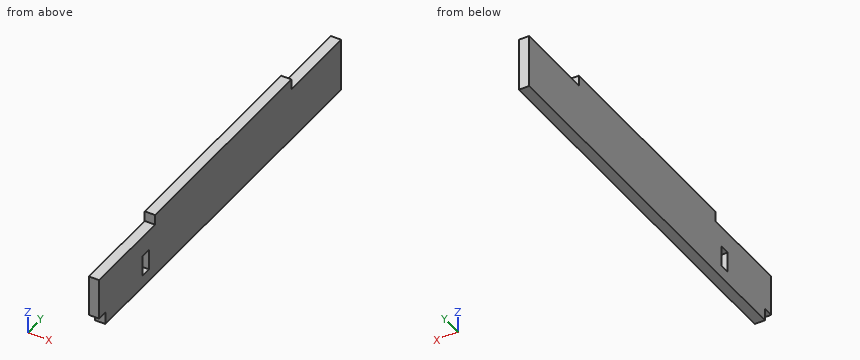
Autodesk Inventor part; units mm, degrees
ref_plane "YZ Plane" through (0, 0, 0) normal (1, 0, 0) x (0, 1, 0)
ref_plane "XZ Plane" through (0, 0, 0) normal (0, 1, 0) x (-1, 0, 0)
ref_plane "XY Plane" through (0, 0, 0) normal (0, 0, 1) x (1, 0, 0)
sketch "Sketch1" plane through (0, 0, 0) normal (1, 0, 0) x (0, 1, 0)
  line L0 (0, 0) -> (200, 0)
  line L1 (200, 0) -> (200, 31)
  line L2 (200, 31) -> (0, 31)
  line L3 (0, 31) -> (0, 0)
  dimension "d0" = 31
  dimension "d1" = 200
extrude "Extrusion1" add sketch "Sketch1" along normal blind 5
sketch "Sketch2" plane through (0, 0, 0) normal (-1, 0, 0) x (0, 0, 1)
  line L0 (0, 200) -> (31, 200)
  line L1 (31, 200) -> (26, 200)
  line L2 (26, 200) -> (26, 195)
  line L3 (26, 195) -> (31, 195)
  line L4 (31, 195) -> (31, 200)
  line L5 (0, 200) -> (5, 200)
  line L6 (5, 200) -> (5, 195)
  line L7 (5, 195) -> (0, 195)
  line L8 (0, 195) -> (0, 200)
  line L9 (31, 0) -> (0, 0)
  line L10 (0, 0) -> (5, 0)
  line L11 (5, 0) -> (5, 5)
  line L12 (5, 5) -> (0, 5)
  line L13 (0, 5) -> (0, 0)
  line L14 (31, 200) -> (31, 0)
  line L15 (31, 0) -> (26, 0)
  line L16 (26, 0) -> (26, 5)
  line L17 (26, 5) -> (31, 5)
  line L18 (31, 5) -> (31, 0)
  line L19 (31, 195) -> (26, 195)
  line L20 (26, 195) -> (26, 155)
  line L21 (26, 155) -> (31, 155)
  line L22 (31, 155) -> (31, 195)
  line L23 (31, 5) -> (26, 5)
  line L24 (26, 5) -> (26, 45)
  line L25 (26, 45) -> (31, 45)
  line L26 (31, 45) -> (31, 5)
  point P0 (31, 5)
  point P1 (26, 0)
  point P2 (31, 45)
  point P3 (31, 155)
  dimension "d4" = 5
  dimension "d5" = 5
  dimension "d6" = 5
  dimension "d7" = 5
  dimension "d8" = 5
  dimension "d9" = 5
  dimension "d10" = 5
  dimension "d11" = 5
  dimension "d14" = 40
  dimension "d15" = 40
extrude "Extrusion2" cut sketch "Sketch2" against normal blind 10 contours L0 L4 L3 L2 | L3 L14 L21 L20 | L9 L16 L17 L14 | L17 L24 L25 L14
sketch "Sketch3" plane through (0, 0, 0) normal (-1, 0, 0) x (0, 0, 1)
  line L0 (6, 35) -> (16, 35)
  line L1 (6, 40) -> (16, 40)
  line L2 (1, 40) -> (1, 35)
  line L3 (16, 40) -> (16, 35)
  line L4 (26, 45) -> (26, 0)
  point P0 (0, 0)
  point P1 (26, 0)
sketch "Sketch3 outline for Extrusion3" plane through (0, 0, 0) normal (-1, 0, 0) x (0, 0, 1)
  line L0 (6, 40) -> (6, 35)
  line L1 (16, 40) -> (6, 40)
  line L2 (16, 35) -> (16, 40)
  line L3 (6, 35) -> (16, 35)
extrude "Extrusion3" cut sketch "Sketch3 outline for Extrusion3" against normal blind 10
sketch "Sketch4" plane through (0, 0, 0) normal (-1, 0, 0) x (0, 0, 1)
  line L0 (26, 200) -> (26, 155)
  line L1 (0, 0) -> (0, 200)
  line L2 (26, 200) -> (0, 200)
  line L3 (0, 200) -> (0, 195)
  line L4 (0, 195) -> (26, 195)
  line L5 (26, 195) -> (26, 200)
  dimension "d18" = 5
extrude "Extrusion4" cut sketch "Sketch4" against normal blind 10
sketch "Sketch5" plane through (5, 0, 0) normal (1, 0, 0) x (0, 0, -1)
  line L0 (0, 0) -> (0, 195)
  line L1 (0, 0) -> (-6, 0)
  line L2 (-6, 0) -> (-6, 5)
  line L3 (-6, 5) -> (0, 5)
  line L4 (0, 5) -> (0, 0)
  line L5 (-6, 40) -> (-6, 35)
  point P0 (0, 5)
  dimension "d21" = 6
  dimension "d22" = 5
  dimension "d23" = 6
extrude "Extrusion5" cut sketch "Sketch5" against normal blind 10
equation "\"d6\" = d4"
equation "\"d7\" = d4"
equation "\"d8\" = d5"
equation "\"d9\" = d8"
equation "\"d11\" = d8"
properties part number "FanVerticalPlate"
Design review of the part built by this model. Coordinates are the model's own, in mm. Coordinates: 2 decimals unless noted, no trailing zeros. Order: outer loops, then holes, each group sorted by start corner. A loop starts at its lowest first (then second) coordinate and runs counter-clockwise, first axis right, second up. Notation, with made-up numbers: M 83.25,-35.75 L 114.25,-35.75 A33 ccw 114.25,-0.75 Z; hole C 43,-20 d10. An arc over 180 degrees is marked long. Answer as a JSON object with one key per item and string values. Group by question number.
1) Add section C-C, the plane y = 181.5. Write out the cut boundary in (x, z), then the cut area to 3 significant figures.
2) Add section B-B, the plane z = 11.5. Write out the cut boundary in (x, y).
3) Add section A-A, the plane x = 1.45. Write out the cut boundary in (y, z).
4) Wall thickness on L1, parallel to Y at x = 3.4, z = 12; L2, parallel to Z at x = 2.2, y = 39; L3, parallel to Z at x = 3.55, y = 167.5: over which ranges is each line inside the solid? List them lowest first.
5) For pin 1 (2.5 mm diameter, centred on x = 2.5, y = 166.5, fed in from +Z); pin 2 (3 mm diameter, centred on y = 36, z = 20.5, fed in from -X); pin 3 (2.5 mm diameter, centred on x = 3.5, y = 2.5, fed in from -Z); pin 4 (1.5 mm diameter, centred on x = 2.5, z = 4, fed in from -Y), all flat-tipped, find the tip position at first contact; note any pin that passes through.
Computed values:
{
 "1": {"outline": "M 0,0 L 5,0 L 5,26 L 0,26 Z", "area": "130 mm^2"},
 "2": {"outline": "M 0,0 L 5,0 L 5,35 L 0,35 Z; M 0,40 L 5,40 L 5,195 L 0,195 Z"},
 "3": {"outline": "M 0,6 L 5,6 L 5,0 L 195,0 L 195,26 L 155,26 L 155,31 L 45,31 L 45,26 L 0,26 Z; hole M 35,6 L 40,6 L 40,16 L 35,16 Z"},
 "4": {"L1": "y = 0 to 35, 40 to 195", "L2": "z = 0 to 6, 16 to 26", "L3": "z = 0 to 26"},
 "5": {"pin 1": "stops at z = 26", "pin 2": "stops at x = 0", "pin 3": "stops at z = 6", "pin 4": "stops at y = 5"}
}
